Check sheet for the modelled part. Datum: model origin and axes. Units: mm. A direction names the side the tool comes from. Coordinates: 2 decimals unless noted, no trailing zeros. Loops run counter-clockwise (first coordinate to the right, second up) from the corner with the lowest first, then second, coordinate; pieces in that order, holes last. Notation, with made-up numbers: (-14, -27.5) - (18, -27.5) arc R18 cw to (18, -2.5) - close; hole circle Ø8 at (66.5, 78.5). An arc over 180 degrees is marked (long way). Use a Markdown table: item, result. Add a question column.
1) Sectioned sample at C-C, the plane z = -12.5. Enter the section's corners in (x, y).
2) Thickness scan on line 1 (X direction, y = 5.5, z = -1.5); line 2 (X direction, y = -7, z = -15.75); line 3 (Y direction, x = 6, z = -20.25). Record the ranges inside material, lowest first.
3) Draft check along X on faces 5 (the flat face through (-27, 0, -21)), 6 (the flat face through (14, 25, -12)), 7 (the flat face through (-25, 20, -12)). Enter one of: pulls with the +X half, pulls with the -X half, needs draft (parallel to the pull), parting line crosses it, or undercut.
4) Go/stop test with flat-tipped pins: P1, Ø10.5, axis at x = -27, z = -7.5, coming from the +Y side; P2, Ø6, axis at x = -25, z = -10.5, coming from the -Y side; P3, Ø3, axis at x = -24, z = -5.5, coming from the -Y side. Record where each tip stops, or that it passes through.
5) Sectioned sample at A-A, the plane y = 0. Enter the section's corners in (x, z).
6) Tool access check on faces 1 (the flat face through (-33, -2, -22)), 2 (the cylindrical face through (-14.87, 29.61, -12.68)), 3 (the flat face through (-27, -6.5, -10)), 4 (the flat face through (-31, 0, -23)). Record the directions out of +Z, -Z, +X, -X, +Y, -Y that give a thin tool (end or side, any length) a straight path to the whole face; none if there is none.
7) Sectioned sample at B-B, the plane z = -22.25. Enter the section's corners in (x, y).
8) Sectioned sample at D-D, the plane x = 1. Enter the section's corners in (y, z).
from build123d import *

# Parameters (mm, degrees)
F0_W     = 54
F0_H     = 60
F0_W_2   = 13
F0_H_2   = 13
F0_W_3   = 14
F0_H_3   = 46
F1_DEPTH = 25
F2_DEPTH = 21
F3_DEPTH = 23
F5_DEPTH = 4
F6_SIZE  = 20
F7_SIZE  = 20
F8_SIZE  = 10
F9_R     = 5


with BuildPart() as f1:
    # F0 (on Top) → F1 (new body)
    with BuildSketch(Plane.XY):
        with Locations((-8, 0)):
            Rectangle(F0_W, F0_H)
        with Locations((-26.8, 0)):
            Rectangle(F0_W_2, F0_H_2, mode=Mode.SUBTRACT)
        Rectangle(F0_W_3, F0_H_3, mode=Mode.SUBTRACT)
        with Locations((-26.8, 0)):
            Rectangle(F0_W_2, F0_H_2)
        Rectangle(F0_W_3, F0_H_3)
    extrude(amount=-F1_DEPTH)

    # F0 (on Top) → F2 (cut)
    with BuildSketch(Plane.XY):
        with Locations((-26.8, 0)):
            Rectangle(F0_W_2, F0_H_2)
    extrude(amount=-F2_DEPTH, mode=Mode.SUBTRACT)

    # F0 (on Top) → F3 (cut)
    with BuildSketch(Plane.XY):
        Rectangle(F0_W_3, F0_H_3)
    extrude(amount=-F3_DEPTH, mode=Mode.SUBTRACT)

    # F4 (on face) → F5 (cut)
    with BuildSketch(Plane(origin=(-35, 0, 0), x_dir=(0, -1, 0), z_dir=(-1, 0, 0))):
        with BuildLine():
            Line((-2, -25), (2, -25))
            Line((2, -25), (2, -17))
            ThreePointArc((2, -17), (0, -19), (-2, -17))
            Line((-2, -17), (-2, -25))
        make_face()
        with BuildLine():
            ThreePointArc((-2, -17), (0, -19), (2, -17))
            Line((2, -17), (-2, -17))
        make_face()
        with BuildLine():
            Line((-2, -17), (2, -17))
            ThreePointArc((2, -17), (0, -15), (-2, -17))
        make_face()
    extrude(amount=-F5_DEPTH, mode=Mode.SUBTRACT)

    # F6
    f6_edges = [f1.edges().sort_by_distance(p)[0] for p in [
        (-35, 30, -12.5),
    ]]
    chamfer(f6_edges, length=F6_SIZE)

    # F7
    f7_edges = [f1.edges().sort_by_distance(p)[0] for p in [
        (-35, -30, -12.5),
    ]]
    chamfer(f7_edges, length=F7_SIZE)

    # F8
    f8_edges = [f1.edges().sort_by_distance(p)[0] for p in [
        (19, -30, -12.5),
        (19, 30, -12.5),
    ]]
    chamfer(f8_edges, length=F8_SIZE)

    # F9
    f9_edges = [f1.edges().sort_by_distance(p)[0] for p in [
        (-35, 10, -12.5),
        (-35, -10, -12.5),
        (-15, -30, -12.5),
        (9, -30, -12.5),
        (19, -20, -12.5),
        (19, 20, -12.5),
        (9, 30, -12.5),
        (-15, 30, -12.5),
    ]]
    fillet(f9_edges, radius=F9_R)


solid = f1.part
Solved:
| question | item | result |
|---|---|---|
| 1 | outline | (-35, -7.93) arc R5 ccw to (-33.54, -11.46) - (-16.46, -28.54) arc R5 ccw to (-12.93, -30) - (6.93, -30) arc R5 ccw to (10.46, -28.54) - (17.54, -21.46) arc R5 ccw to (19, -17.93) - (19, 17.93) arc R5 ccw to (17.54, 21.46) - (10.46, 28.54) arc R5 ccw to (6.93, 30) - (-12.93, 30) arc R5 ccw to (-16.46, 28.54) - (-33.54, 11.46) arc R5 ccw to (-35, 7.93) - close; hole (-33.3, -6.5) - (-20.3, -6.5) - (-20.3, 6.5) - (-33.3, 6.5) - close; hole (-7, -23) - (7, -23) - (7, 23) - (-7, 23) - close |
| 2 | line 1 | x = -35 to -33.3, -20.3 to -7, 7 to 19 |
| 2 | line 2 | x = -35 to -7, 7 to 19 |
| 2 | line 3 | y = -30 to -23, 23 to 30 |
| 3 | face 5 | undercut |
| 3 | face 6 | pulls with the +X half |
| 3 | face 7 | pulls with the -X half |
| 4 | P1 | stops at y = 23.25 |
| 4 | P2 | stops at y = -23 |
| 4 | P3 | stops at y = -22.5 |
| 5 | outline | (-35, -15) - (-33.3, -15) - (-33.3, 0) - (-35, 0) - close; (-31, -25) - (19, -25) - (19, 0) - (7, 0) - (7, -23) - (-7, -23) - (-7, 0) - (-20.3, 0) - (-20.3, -21) - (-31, -21) - close |
| 6 | face 1 | -Z, -X |
| 6 | face 2 | +Z, -Z, -X, +Y |
| 6 | face 3 | +Z |
| 6 | face 4 | +Z, -Z, -X |
| 7 | outline | (-35, -7.93) arc R5 ccw to (-33.54, -11.46) - (-16.46, -28.54) arc R5 ccw to (-12.93, -30) - (6.93, -30) arc R5 ccw to (10.46, -28.54) - (17.54, -21.46) arc R5 ccw to (19, -17.93) - (19, 17.93) arc R5 ccw to (17.54, 21.46) - (10.46, 28.54) arc R5 ccw to (6.93, 30) - (-12.93, 30) arc R5 ccw to (-16.46, 28.54) - (-33.54, 11.46) arc R5 ccw to (-35, 7.93) - (-35, 2) - (-31, 2) - (-31, -2) - (-35, -2) - close; hole (-7, -23) - (7, -23) - (7, 23) - (-7, 23) - close |
| 8 | outline | (-30, -25) - (30, -25) - (30, 0) - (23, 0) - (23, -23) - (-23, -23) - (-23, 0) - (-30, 0) - close |
